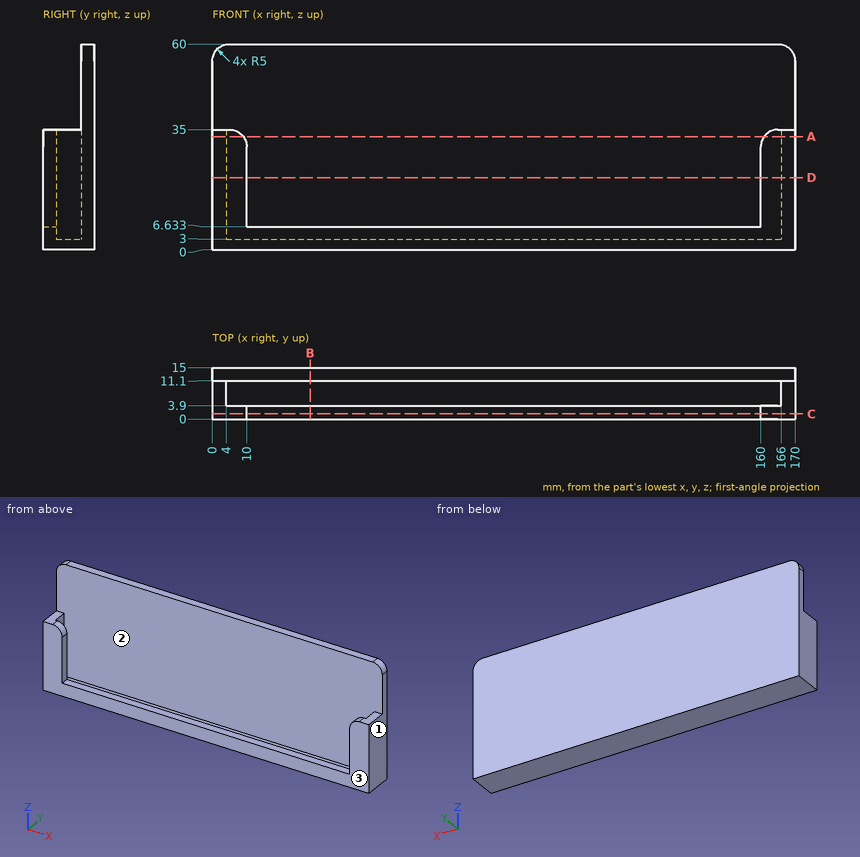
For this review, use the dimensioned drawing (mm, ordinates from the lowest corner) and the shaded views. Give positions to 0.01 mm unless a question says otherwise; leave off trailing zeros. Write each loop counter-clockwise with the first axis right and the second up, starting at its lowest first coordinate (ties: lowest second). Pieces come first, ordered by that corner, then holes.
(1) To check wall thickness, follow L1, parallel to X at y = 3, z = 20.5; L2, parallel to X at y = 7.75, z = 29.5; L3, parallel to Z at x = 24, y = 5. State the ranges of each line that lie inside material, in increasing order.
(2) For P1, Ø3, axis at x = 116, z = 28.5, coming from the -Y side; P2, Ø5.5, axis at x = 2, y = 3, coming from the +Z side; P3, Ø4.5, axis at x = 53, y = 2, coming from the +Z side, all flat-tipped, find the tip position at first contact; note any pin that passes through.
(3) The part is to be moulded in two halves that separate along X. For the marked faces 1, 2 and 3, say which applies: released by +X, released by -X, zero draft, split by the parting line, or undercut.
(4) Consider section C-C, the plane y = 1.5. Give the boundary of the cut face in (x, z), and give its area (3 significant figures).
(5) Consider section A-A, the plane z = 33. Give the boundary of the cut face in (x, y).
(6) Consider section D-D, the plane z = 21. Give the boundary of the cut face in (x, y).
(7) Consider section B-B, the plane x = 28.5. Give the boundary of the cut face in (y, z).
Returned:
1. L1: x = 0 to 10, 160 to 170
1. L2: x = 0 to 4, 166 to 170
1. L3: z = 0 to 3
2. P1: stops at y = 11.1
2. P2: stops at z = 35
2. P3: stops at z = 6.63
3. face 1: released by +X
3. face 2: undercut
3. face 3: zero draft
4. outline: (0, 0) - (170, 0) - (170, 35) - (165, 35) arc R5 ccw to (160, 30) - (160, 6.63) - (10, 6.63) - (10, 30) arc R5 ccw to (5, 35) - (0, 35) - close
4. area: 1,680 mm2
5. outline: (0, 0) - (9, 0) - (9, 3.9) - (4, 3.9) - (4, 11.1) - (166, 11.1) - (166, 3.9) - (161, 3.9) - (161, 0) - (170, 0) - (170, 15) - (0, 15) - close
6. outline: (0, 0) - (10, 0) - (10, 3.9) - (4, 3.9) - (4, 11.1) - (166, 11.1) - (166, 3.9) - (160, 3.9) - (160, 0) - (170, 0) - (170, 15) - (0, 15) - close
7. outline: (0, 0) - (15, 0) - (15, 60) - (11.1, 60) - (11.1, 3) - (3.9, 3) - (3.9, 6.63) - (0, 6.63) - close
